Autodesk Inventor part; units mm, degrees
ref_plane "Work Plane1" through (2.54, 9.35, 0) normal (0, 1, 0) x (1, 0, 0)
ref_plane "YZ Plane" through (0, 0, 0) normal (1, 0, 0) x (0, 1, 0)
ref_plane "XZ Plane" through (0, 0, 0) normal (0, 1, 0) x (-1, 0, 0)
sketch "Sketch1" plane through (0, 0, 0) normal (0, 1, 0) x (-1, 0, 0)
  circle A0 centre (0, 0) radius 0.4191
  circle A1 centre (2.54, 0) radius 0.4191
  circle A2 centre (-2.54, 0) radius 0.4191
  dimension "d0" = 0.8382
  dimension "d1" = 0.8382
  dimension "d2" = 0.8382
  dimension "d3" = 2.54
  dimension "d4" = 2.54
extrude "Extrusion1" add sketch "Sketch1" along normal blind 11
ref_plane "Work Plane1" through (2.54, 9.35, 0) normal (0, 1, 0) x (1, 0, 0)
sketch "Sketch2" plane through (2.54, 9.35, 0) normal (0, 1, 0) x (1, 0, 0)
  line L0 (-6.35, 1.27) -> (1.27, 1.27)
  line L1 (1.27, 1.27) -> (1.27, -1.27)
  line L2 (1.27, -1.27) -> (-6.35, -1.27)
  line L3 (-6.35, -1.27) -> (-6.35, 1.27)
  point P0 (-2.54, 0)
  dimension "d8" = 3.81
  dimension "d9" = 3.81
  dimension "d10" = 1.27
  dimension "d11" = 2.54
extrude "Extrusion2" add sketch "Sketch2" against normal blind 2
properties part number "3PinHeader"
Check sheet for the modelled part. Datum: model origin and axes. Units: mm. A direction names the side the tool comes from. Round coordinates to 2 decimals unless told otherwise and drop trailing zeros. Order: outer loops, then holes, each group sorted by start corner. A loop starts at its lowest first (then second) coordinate and runs counter-clockwise, first axis right, second up.
(1) Cross-section at C-C, the plane z = 0. Enter the section's corners in (x, y).
(2) Access from +Z, -Z, +X, -X, +Y, -Y to the whole of each face (thin tool, end or side, straight path). Record for faces 1 (the flat face through (0, 9.35, 1)), 2 (the flat face through (-2.5, 0, 0)), 3 (the flat face through (0, 7.35, 1)).
(3) Cross-section at A-A, the plane y = 6. Enter the section's corners in (x, z).
(4) Draft check along X on faces 4 (the flat face through (3.81, 8, 0)), 5 (the flat face through (2.5, 11, 0)), 6 (the cylindrical face through (-2.927, 3.624, 0.161)). Enter one of: pulls with the +X half, pulls with the -X half, needs draft (parallel to the pull), parting line crosses it, or undercut.
(5) Scan lines: probe 1 along X at (y, z) = (6.5, -0.2); probe 2 along Y at (x, z) = (0.5, 0.35); probe 3 along Z at (x, y) = (-2.5, 5.75). Record each from-to range of solid material in increasing order.
(6) Cross-section at D-D, the plane z = 1.15. Enter the section's corners in (x, y), and give its area (3 significant figures).
(7) Cross-section at B-B, the plane x = -2.54. Enter the section's corners in (y, z).
Check sheet entries:
1. outline: (-3.81, 7.35) - (-2.96, 7.35) - (-2.96, 0) - (-2.12, 0) - (-2.12, 7.35) - (-0.42, 7.35) - (-0.42, 0) - (0.42, 0) - (0.42, 7.35) - (2.12, 7.35) - (2.12, 0) - (2.96, 0) - (2.96, 7.35) - (3.81, 7.35) - (3.81, 9.35) - (2.96, 9.35) - (2.96, 11) - (2.12, 11) - (2.12, 9.35) - (0.42, 9.35) - (0.42, 11) - (-0.42, 11) - (-0.42, 9.35) - (-2.12, 9.35) - (-2.12, 11) - (-2.96, 11) - (-2.96, 9.35) - (-3.81, 9.35) - close
2. face 1: +Y
2. face 2: +Z, -Z, +X, -X, -Y
2. face 3: -Y
3. outline: circle Ø0.84 at (-2.54, 0); circle Ø0.84 at (0, 0); circle Ø0.84 at (2.54, 0)
4. face 4: pulls with the +X half
4. face 5: needs draft
4. face 6: undercut
5. probe 1: x = -2.91 to -2.17, -0.37 to 0.37, 2.17 to 2.91
5. probe 2: y = 7.35 to 9.35
5. probe 3: z = -0.42 to 0.42
6. outline: (-3.81, 7.35) - (3.81, 7.35) - (3.81, 9.35) - (-3.81, 9.35) - close
6. area: 15.2 mm2
7. outline: (0, -0.42) - (7.35, -0.42) - (7.35, -1.27) - (9.35, -1.27) - (9.35, -0.42) - (11, -0.42) - (11, 0.42) - (9.35, 0.42) - (9.35, 1.27) - (7.35, 1.27) - (7.35, 0.42) - (0, 0.42) - close
